Geometry check sheet. Reference: the model listing, model coordinates, mm. A direction names the side the tool comes from. Round coordinates to 2 decimals unless told otherwise and drop trailing zeros. Write each loop counter-clockwise with the first axis right and the second up, starting at its lowest first coordinate (ties: lowest second). Pieces come first, ordered by that corner, then holes.
from build123d import *

# Parameters (mm, degrees)
F1_DEPTH      = 95
F3_DEPTH      = 150
F3_DEPTH_BACK = 150
F5_DEPTH      = 25


with BuildPart() as f1:
    # F0 (on Right) → F1 (new body)
    with BuildSketch(Plane.YZ):
        Polygon((-87.993201702, 5), (-87.993201702, 0), (162.006798298, 0), (162.006798298, 5), (137.006798298, 5), (87.006798298, 5), (-2.993201702, 5), (-62.993201702, 5), align=None)
        with BuildLine():
            Line((-62.993201702, 35), (-62.993201702, 5))
            Line((-62.993201702, 5), (-2.993201702, 5))
            Line((-2.993201702, 5), (-2.993201702, 27.5))
            ThreePointArc((-2.993201702, 27.5), (-10.493201702, 35), (-2.993201702, 42.5))
            Line((-2.993201702, 42.5), (-2.993201702, 95))
            ThreePointArc((-2.993201702, 95), (-28.3502974065, 89.3784672222), (-48.9558682892, 73.5672565812))
            Line((-48.9558682892, 73.5672565812), (-33.6349794268, 60.7115043875))
            Line((-33.6349794268, 60.7115043875), (-38.4558864994, 54.9661710641))
            Line((-38.4558864994, 54.9661710641), (-53.7767753618, 67.8219232578))
            ThreePointArc((-53.7767753618, 67.8219232578), (-60.6174576688, 55.9735139436), (-62.993201702, 42.5))
            Line((-62.993201702, 42.5), (-42.993201702, 42.5))
            Line((-42.993201702, 42.5), (-42.993201702, 35))
            Line((-42.993201702, 35), (-62.993201702, 35))
        make_face()
        with BuildLine():
            Line((87.006798298, 5), (137.006798298, 5))
            add(Edge.make_bspline(
                [(-2.993201702, 95), (30.6227877736, 95.7361534238), (79.8862645285, 82.5462463817), (121.0056993256, 58.60780489), (133.2323859183, 24.3846146975), (137.006798298, 5)],
                knots=[0, 0, 0, 0, 0.3988693097, 0.6832428088, 1, 1, 1, 1], degree=3))
            Line((-2.993201702, 95), (-2.993201702, 42.5))
            ThreePointArc((-2.993201702, 42.5), (2.3100991569, 40.3033008589), (4.506798298, 35))
            ThreePointArc((4.506798298, 35), (2.3100991569, 29.6966991411), (-2.993201702, 27.5))
            Line((-2.993201702, 27.5), (-2.993201702, 5))
            Line((-2.993201702, 5), (87.006798298, 5))
        make_face()
        with BuildLine():
            ThreePointArc((94.506798298, 40), (92.3100991569, 34.6966991411), (87.006798298, 32.5))
            ThreePointArc((87.006798298, 32.5), (81.7034974391, 45.3033008589), (94.506798298, 40))
        make_face(mode=Mode.SUBTRACT)
    extrude(amount=F1_DEPTH)

    # F2 (on Front) → F3 (cut, two sides)
    with BuildSketch(Plane.XZ) as f3_sk:
        Polygon((5, 5), (90, 5), (90, 95), (90, 99.046766758), (5, 99.046766758), (5, 95), align=None)
    extrude(amount=-F3_DEPTH, mode=Mode.SUBTRACT)
    extrude(f3_sk.sketch, amount=F3_DEPTH_BACK, mode=Mode.SUBTRACT)

    # F4 (on face) → F5 (cut)
    with BuildSketch(Plane(origin=(0, 0, 0), x_dir=(1, 0, 0), z_dir=(0, 0, -1))):
        with BuildLine():
            Line((20, 26.493201702), (20, 27.993201702))
            Line((20, 27.993201702), (21.5, 27.993201702))
            ThreePointArc((21.5, 27.993201702), (18.9393398282, 29.0538618738), (20, 26.493201702))
        make_face()
        with BuildLine():
            Line((21.5, 27.993201702), (20, 27.993201702))
            Line((20, 27.993201702), (20, 26.493201702))
            ThreePointArc((20, 26.493201702), (21.0606601718, 26.9325415303), (21.5, 27.993201702))
        make_face()
        with BuildLine():
            Line((75, 27.993201702), (73.5, 27.993201702))
            ThreePointArc((73.5, 27.993201702), (73.9393398282, 26.9325415303), (75, 26.493201702))
            Line((75, 26.493201702), (75, 27.993201702))
        make_face()
        with BuildLine():
            ThreePointArc((76.5, 27.993201702), (75, 29.493201702), (73.5, 27.993201702))
            Line((73.5, 27.993201702), (75, 27.993201702))
            Line((75, 27.993201702), (75, 26.493201702))
            ThreePointArc((75, 26.493201702), (76.0606601718, 26.9325415303), (76.5, 27.993201702))
        make_face()
        with BuildLine():
            ThreePointArc((21.5, -102.006798298), (21.0606601718, -100.9461381262), (20, -100.506798298))
            Line((20, -100.506798298), (20, -102.006798298))
            Line((20, -102.006798298), (21.5, -102.006798298))
        make_face()
        with BuildLine():
            Line((20, -102.006798298), (20, -100.506798298))
            ThreePointArc((20, -100.506798298), (18.9393398282, -103.0674584697), (21.5, -102.006798298))
            Line((21.5, -102.006798298), (20, -102.006798298))
        make_face()
        with BuildLine():
            Line((75, -102.006798298), (75, -100.506798298))
            ThreePointArc((75, -100.506798298), (73.9393398282, -100.9461381262), (73.5, -102.006798298))
            Line((73.5, -102.006798298), (75, -102.006798298))
        make_face()
        with BuildLine():
            ThreePointArc((76.5, -102.006798298), (76.0606601718, -100.9461381262), (75, -100.506798298))
            Line((75, -100.506798298), (75, -102.006798298))
            Line((75, -102.006798298), (73.5, -102.006798298))
            ThreePointArc((73.5, -102.006798298), (75, -103.506798298), (76.5, -102.006798298))
        make_face()
    extrude(amount=-F5_DEPTH, mode=Mode.SUBTRACT)


solid = f1.part
1. Section check A-A (x = 59.5). Record the cut outline in (y, z).
2. Release check for a two-part mould opening along X. For faces 1 (the face through (2.46, -36.01, 57.88)), 2 (the face through (0, 35, 38)), 3 (the face through (5, 38, 41)) record: +X half, -X half, draft (parallel to the pull), parting line (faces both ways), or undercut.
3. Access from +Z, -Z, +X, -X, +Y, -Y to the whole of each face (thin tool, end or side, straight path). Record for faces 4 (the face through (92.465, -46.009, 61.304)), 5 (the face through (47, 35, 0)), 6 (the face through (92, -62.993, 20)), 7 (the face through (2, -53, 42.5)).
4. Section check C-C (z = 39). State how many separate pieces and enclosed holes the cut face has, plus the area to 3 significant figures.
5. Depth check by flat-ended pin: pin 1 Ø3.5 at (x, y) = (20, -27.99) entering from -Z; pin 2 Ø2 at (x, y) = (85, 77.5) entering from +Z; pin 3 Ø1.5 at (x, z) = (3, 39.5) entering from -Y; pin 4 Ø4 at (x, y) = (2.5, -48.5) entering from +Z. Enter the tip coordinate at first touch or a pass-through.
6. Section check B-B (y = -13). Record the cut outline in (x, z), plus the area to 3 significant figures.
7. Scan lines: line 1 along X through (y, z) = (42, 61); line 2 along Y through (x, z) = (3, 40); line 3 along Z through (x, y) = (67, -68). Record each from-to range of solid material in increasing order.
Results below:
1. outline: (-87.99, 0) - (162.01, 0) - (162.01, 5) - (-87.99, 5) - close
2. face 1: draft
2. face 2: -X half
2. face 3: undercut
3. face 4: +X, -X
3. face 5: -Z, +X, -X, +Y, -Y
3. face 6: +Z, +X, -X, -Y
3. face 7: +X, -X, -Y
4. separate pieces: 6
4. enclosed holes: 0
4. area: 1,420 mm2
5. pin 1: stops at z = 0
5. pin 2: stops at z = 5
5. pin 3: stops at y = -42.99
5. pin 4: stops at z = 76.32
6. outline: (0, 0) - (95, 0) - (95, 94.16) - (90, 94.16) - (90, 5) - (5, 5) - (5, 94.16) - (0, 94.16) - close
6. area: 1,370 mm2
7. line 1: x = 0 to 5, 90 to 95
7. line 2: y = -42.99 to -8.58, 2.6 to 79.51, 94.51 to 126.02
7. line 3: z = 0 to 5
